Autodesk Inventor part; units mm, degrees
ref_plane "YZ Plane" through (0, 0, 0) normal (1, 0, 0) x (0, 1, 0)
ref_plane "XZ Plane" through (0, 0, 0) normal (0, 1, 0) x (-1, 0, 0)
ref_plane "XY Plane" through (0, 0, 0) normal (0, 0, 1) x (1, 0, 0)
sketch "Sketch1" plane through (0, 0, 0) normal (0, 1, 0) x (-1, 0, 0)
  line L0 (0, 0) -> (6.35, 0)
  line L1 (6.35, 0) -> (6.35, -22.86)
  line L2 (6.35, -22.86) -> (0, -22.86)
  line L3 (0, -22.86) -> (0, 0)
  line L4 (0, 0) -> (3.175, 0)
  line L5 (3.175, 0) -> (3.175, -3.175)
  line L6 (3.175, -3.175) -> (0, -3.175)
  line L7 (0, -3.175) -> (0, 0)
  line L8 (0, -22.86) -> (3.175, -22.86)
  line L9 (3.175, -22.86) -> (3.175, -19.685)
  line L10 (3.175, -19.685) -> (0, -19.685)
  line L11 (0, -19.685) -> (0, -22.86)
  dimension "d0" = 6.35
  dimension "d1" = 22.86
  dimension "d2" = 3.175
  dimension "d3" = 3.175
  dimension "d4" = 3.175
  dimension "d5" = 3.175
extrude "Extrusion1" add sketch "Sketch1" along normal blind 3.175
hole "Hole1" at (-3.175, 0, -3.175) at (-3.175, 0, -19.685) direction (0, 1, 0) diameter 2.7051 depth 6.35
sketch "Sketch2" plane through (0, 0, 0) normal (1, 0, 0) x (0, 0, -1)
  line L0 (0, 3.175) -> (22.86, 3.175)
  circle A0 centre (11.43, 3.175) radius 5.08
  circle A1 centre (11.43, 8.255) radius 2.54
  point P0 (0, 0)
  point P1 (13.8893, 7.62)
  point P2 (8.9707, 7.62)
  point P3 (6.35, 3.175)
  point P4 (16.51, 3.175)
  dimension "d15" = 10.16
  dimension "d16" = 5.08
extrude "Extrusion2" add sketch "Sketch2" against normal blind 6.35 contours A0 A1 L0 | L0 A0
fillet "Fillet1" radius 3.175 2 edges at (0, 5.715, -11.43) (-6.35, 5.715, -11.43)
properties part number "DualSensorReadout - CableClamp"
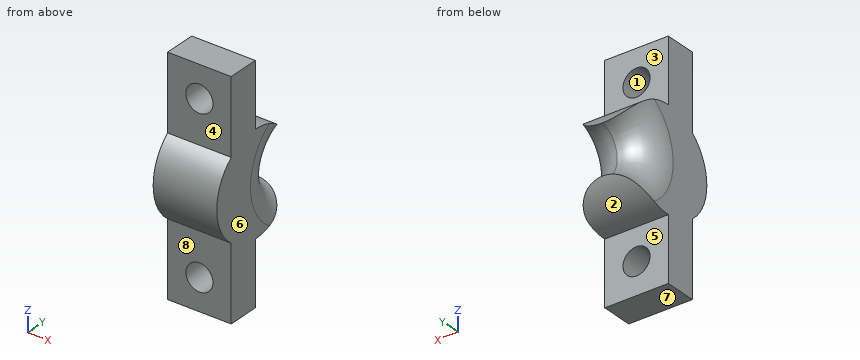
Read the model definition and answer for the solid it produces. Units are mm, in the model's axes. Face numbers are marked on the shaded views. A direction names the side the tool comes from. Give positions to 0.01 mm unless a question says otherwise; leave off trailing zeros. Write each loop counter-clockwise with the first axis right and the second up, starting at its lowest first coordinate (ties: lowest second). Pieces come first, ordered by that corner, then holes. Notation, with made-up numbers: (21.5, 82) -> (30.5, 82) arc R9 ccw to (30.5, 88) -> close; hole circle Ø6 at (30.25, -16.75). An arc over 180 degrees is marked (long way). Answer in a Markdown table with one row per item.
1) Section C-C on y = 2 is taken. Give the vertices of the cut face in (x, z) (3 decimals).
Results list:
| item | result |
|---|---|
| outline | (-6.35, -22.86) -> (0, -22.86) -> (0, 0) -> (-6.35, 0) -> close; hole circle Ø2.705 at (-3.175, -19.685); hole circle Ø2.705 at (-3.175, -3.175) |
2) Each of these flat-tipped pins is pushed along its axis until it touches: pin 1 Ø3 at (x, z) = (-3, -20.5) entering from +Y (3 decimals); pin 2 Ø3 at (x, z) = (-4, -4) entering from -Y; pin 3 Ø1.5 at (x, z) = (-5, -14) entering from -Y; pin 4 Ø2.5 at (x, z) = (-3.175, -19.685) entering from -Y. Where does it stop, or does it pass through?
Results list:
| item | result |
|---|---|
| pin 1 | y = 3.175 |
| pin 2 | y = 0 |
| pin 3 | y = -1.57 |
| pin 4 | through |
3) Section A-A on x = -3.5 is taken. Give the vertices of the cut face in (y, z) (3 decimals), plus the area to 3 significant figures.
Results list:
| item | result |
|---|---|
| outline | (0, -22.86) -> (3.175, -22.86) -> (3.175, -20.998) -> (0, -20.998) -> close; (0, -18.372) -> (3.175, -18.372) -> (3.175, -16.51) arc R5.08 ccw to (7.612, -13.904) arc R2.557 cw to (7.612, -8.956) arc R5.08 ccw to (3.175, -6.35) -> (3.175, -4.488) -> (0, -4.488) -> (0, -7.464) arc R5.08 ccw to (0, -15.396) -> close; (0, -1.862) -> (3.175, -1.862) -> (3.175, 0) -> (0, 0) -> close |
| area | 97.8 mm^2 |
4) Section B-B on z = -2.5 is taken. Give the vertices of the cut face in (x, y) (3 decimals).
Results list:
| item | result |
|---|---|
| outline | (-6.35, 0) -> (-4.347, 0) -> (-4.347, 3.175) -> (-6.35, 3.175) -> close; (-2.003, 0) -> (0, 0) -> (0, 3.175) -> (-2.003, 3.175) -> close |
5) Determine the mould class of the marked faces 1, 2 and 3 for opening direction Z: released by +Z, released by -Z, zero draft, split by the parting line, or undercut.
Results list:
| item | result |
|---|---|
| face 1 | undercut |
| face 2 | released by -Z |
| face 3 | zero draft |
6) Straight lines are drawn through the part: line 1 (Z direction, x = -2, y = 1.75); line 2 (Y direction, x = -1.75, z = -4.75) (3 decimals); line 3 (Z direction, x = -1, y = 6). For each, find the intervals that lie inside material, in ascending order. Write a range as [from, to].
Results list:
| item | result |
|---|---|
| line 1 | [-22.86, -20.35], [-19.02, -3.84], [-2.51, 0] |
| line 2 | [0, 3.175] |
| line 3 | [-15.65, -13.98], [-8.88, -7.21] |
7) Section D-D on z = -21.25 is taken. Give the vertices of the cut face in (x, y) (3 decimals), plus the area to 3 significant figures.
Results list:
| item | result |
|---|---|
| outline | (-6.35, 0) -> (0, 0) -> (0, 3.175) -> (-6.35, 3.175) -> close |
| area | 20.2 mm^2 |
8) A tool of negligible diameter and unlimited length cuts with its end or side. For the marked faces 4, 5, 6, 7 and 8, from which of +Z, -Z, +X, -X, +Y, -Y can it reach the whole face along a straight path? Write none if from no direction.
Results list:
| item | result |
|---|---|
| face 4 | +Z, +X, -X, -Y |
| face 5 | -Z, +X, -X, +Y |
| face 6 | +Z, -Z, +X, +Y, -Y |
| face 7 | -Z, +X, -X, +Y, -Y |
| face 8 | -Z, +X, -X, -Y |
